```python
from build123d import *

# Parameters (mm, degrees)
F0_W     = 50.953738
F0_H     = 51.374846
F1_DEPTH = 25.4
F2_R     = 5.08
F3_SIZE  = 5.08
F4_R     = 9.694572
F5_DEPTH = 25.4


with BuildPart() as f1:
    # F0 (on Front) → F1 (new body)
    with BuildSketch(Plane.XZ):
        Rectangle(F0_W, F0_H)
    extrude(amount=F1_DEPTH)

    # F2
    f2_edges = [f1.edges().sort_by_distance(p)[0] for p in [
        (0, -25.4, 25.687423),
        (25.476869, -25.4, 0),
        (0, -25.4, -25.687423),
        (-25.476869, -25.4, 0),
    ]]
    fillet(f2_edges, radius=F2_R)

    # F3
    f3_edges = [f1.edges().sort_by_distance(p)[0] for p in [
        (0, 0, 25.687423),
        (-25.476869, 0, 0),
        (0, 0, -25.687423),
        (25.476869, 0, 0),
    ]]
    chamfer(f3_edges, length=F3_SIZE)

    # F4 (on face) → F5 (cut)
    with BuildSketch(Plane.XZ.offset(25.4)):
        Circle(F4_R)
    extrude(amount=-F5_DEPTH, mode=Mode.SUBTRACT)


solid = f1.part
```
Part model, mm, in its own coordinate system. Round coordinates to 2 decimals unless told otherwise and drop trailing zeros. Write each loop counter-clockwise with the first axis right and the second up, starting at its lowest first coordinate (ties: lowest second). Pieces come first, ordered by that corner, then holes. Notation, with made-up numbers: (-33, 89.5) -> (-1, 89.5) arc R18 cw to (-1, 102.5) -> close; hole circle Ø1 at (10, -39). An arc over 180 degrees is marked (long way). Return JSON: item names as keys, results as strings. Group by question number.
Q1. Mould opens along Z. For faces 1 (the cylindrical face through (-7.69, -12.88, -5.9)), 2 (the flat face through (-9, -25.4, 5)), 3 (the cylindrical face through (0.36, -23.87, 24.24)) say: pulls with the +Z half, pulls with the -Z half, needs draft (parallel to the pull), parting line crosses it, or undercut.
Q2. Saw through at B-B on x = 0. Write the cut outline in (y, z).
Q3. Saw through at C-C on y = -8. Write the cut outline in (x, z).
Q4. Probe L1, parallel to Z at x = 0, y = -18; L2, parallel to Z at x = -1, y = -9.75; L3, parallel to Z at x = 21.5, y = -21.75. List the from-to ranges inside material, lowest first. Write a range as [from, to].
Q5. Saw through at A-A on z = 0. Write the cut outline in (x, y), plus the area to 3 significant figures.
Q6. Saw through at D-D on z = 18. Write the cut outline in (x, y).
Answer:
{
 "1": {"face 1": "undercut", "face 2": "needs draft", "face 3": "pulls with the +Z half"},
 "2": {"outline": "(-25.4, -20.61) arc R5.08 ccw to (-20.32, -25.69) -> (-5.08, -25.69) -> (0, -20.61) -> (0, -9.69) -> (-25.4, -9.69) -> close; (-25.4, 9.69) -> (0, 9.69) -> (0, 20.61) -> (-5.08, 25.69) -> (-20.32, 25.69) arc R5.08 ccw to (-25.4, 20.61) -> close"},
 "3": {"outline": "(-25.48, -25.69) -> (25.48, -25.69) -> (25.48, 25.69) -> (-25.48, 25.69) -> close; hole circle Ø19.39 at (0, 0)"},
 "4": {"L1": "[-25.69, -9.69], [9.69, 25.69]", "L2": "[-25.69, -9.64], [9.64, 25.69]", "L3": "[-25.48, 25.48]"},
 "5": {"outline": "(-25.48, -20.32) arc R5.08 ccw to (-20.4, -25.4) -> (-9.69, -25.4) -> (-9.69, 0) -> (-20.4, 0) -> (-25.48, -5.08) -> close; (9.69, -25.4) -> (20.4, -25.4) arc R5.08 ccw to (25.48, -20.32) -> (25.48, -5.08) -> (20.4, 0) -> (9.69, 0) -> close", "area": "765 mm2"},
 "6": {"outline": "(-25.48, -20.32) arc R5.08 ccw to (-20.4, -25.4) -> (20.4, -25.4) arc R5.08 ccw to (25.48, -20.32) -> (25.48, -5.08) -> (20.4, 0) -> (-20.4, 0) -> (-25.48, -5.08) -> close"}
}
